```python
from build123d import *

# Parameters (mm, degrees)
CHAMFER1_SIZE = 0.5
FILLET1_R     = 10


with BuildPart() as part:
    # Sketch1 → Revolve1 (revolve)
    with BuildSketch(Plane(origin=(0, 0, 0), x_dir=(0, 0, -1), z_dir=(1, 0, 0)), mode=Mode.PRIVATE) as revolve1_sk:
        Polygon((0, 0), (0, -80), (11.00000000000001, -80), (11.00000000000001, -77), (2.5000000000000098, -77), (2.5000000000000098, -8), (1.4957064412197685, -8), (1.4957064412197685, -3.000000000000001), (2.500000000000019, -3.000000000000001), (2.500000000000019, -4e-16), align=None)
    revolve(revolve1_sk.sketch.rotate(Axis((0, 0, 0), (0, -1, 0)), 180), axis=Axis((0, 0, 0), (0, -1, 0)))

    # Chamfer1
    chamfer1_edges = [part.edges().sort_by_distance(p)[0] for p in [
        (-6.1e-16, -4e-16, -2.500000000000019),
    ]]
    chamfer(chamfer1_edges, length=CHAMFER1_SIZE)

    # Fillet1
    # the kernel refuses this fillet: 10 mm, written as the material it adds along each edge
    with BuildSketch(Plane(origin=(0, -77, 0), x_dir=(1.2e-16, 0, 1), z_dir=(1, 0, -1.2e-16))) as fillet1_piece_1:
        with BuildLine():
            CenterArc((12.500000000000007, -9.886859966642888), FILLET1_R, 98.62692655867836, 81.37307344132165)
            Line((11.000000000000053, -2.8422e-13), (10.970000000000054, 0.19773719933256473))
            ThreePointArc((10.970000000000054, 0.19773719933256473), (6.750000000000032, 0.20000000000000284), (2.5000000000000098, 0.20000000000000284))
            Line((2.5000000000000098, 0.20000000000000284), (2.3000000000000096, 0))
            Line((2.3000000000000096, 0), (2.300000000000007, -9.886859966642888))
            Line((2.300000000000007, -9.886859966642888), (2.500000000000007, -9.886859966642888))
        make_face()
    revolve(axis=Axis((0, -77, 0), (0, -1, 0)))


solid = part.part
```
Can you work these out from the model? Positions are in its coordinate system, mm. A direction names the side the tool comes from. Coordinates: 2 decimals unless noted, no trailing zeros. Order: outer loops, then holes, each group sorted by start corner. A loop starts at its lowest first (then second) coordinate and runs counter-clockwise, first axis right, second up.
1. I'm going to push flat-ended pins straight in: pin 1 (12 mm diameter, centred on y = -56.5, z = 0, fed in from -X); pin 2 (10 mm diameter, centred on x = -0.5, z = -8.5, fed in from +Y); pin 3 (6 mm diameter, centred on y = -69.5, z = -8, fed in from +X); pin 4 (4 mm diameter, centred on y = -34, z = -1.5, fed in from +X). Where does each tip first touch, or does it pass through?
2. Thinking about a two-plate mould opening in Y: for faces 1 (the face through (0, -80, 0)), 2 (the face through (-1.69, -1.73, -1.84)), 3 (the face through (2, -8, 0)), which applies, +Y half, -Y half, draft (parallel to the pull), parting line (faces both ways), or undercut?
3. I need wall thicknesses on line 1 (Y direction, x = 0, z = -1.75); line 2 (X direction, y = -23, z = -0.25); line 3 (Y direction, x = 6.5, z = -6.5). Which ranges of each line are inside material? Lowest first, please.
4. If we section it at B-B (x = 0): Please give me the cut outline in (y, z).
5. If we section it at A-A (z = 0): Please give me the cut outline in (x, y), then the cut area to 3 significant figures.
6. If we section it at D-D (y = -74.5): Please give me the cut outline in (x, z), then the cut area to 3 significant figures.
7. If we section it at C-C (y = -6): Please give me the cut outline in (x, z).
8. For faces 4 (the face through (0, 0, 0)), 5 (the face through (1.46, -5.46, -0.32)), 6 (the face through (2.44, -37.14, -0.54)), which set-ups out of +Z, -Z, +X, -X, +Y, -Y let a thin tool reach every point of the face, with its end or its side?
Entries:
1. pin 1: stops at x = -2.5
1. pin 2: stops at y = -71.5
1. pin 3: passes through
1. pin 4: stops at x = 2.5
2. face 1: -Y half
2. face 2: draft
2. face 3: undercut
3. line 1: y = -80 to -8, -3 to 0
3. line 2: x = -2.49 to 2.49
3. line 3: y = -80 to -76.55
4. outline: (-80, -11) - (-77, -11) arc R10 cw to (-67.11, -2.5) - (-8, -2.5) - (-8, -1.5) - (-3, -1.5) - (-3, -2.5) - (-0.5, -2.5) - (0, -2) - (0, 2) - (-0.5, 2.5) - (-3, 2.5) - (-3, 1.5) - (-8, 1.5) - (-8, 2.5) - (-67.11, 2.5) arc R10 cw to (-77, 11) - (-80, 11) - close
5. outline: (-11, -80) - (11, -80) - (11, -77) arc R10 cw to (2.5, -67.11) - (2.5, -8) - (1.5, -8) - (1.5, -3) - (2.5, -3) - (2.5, -0.5) - (2, 0) - (-2, 0) - (-2.5, -0.5) - (-2.5, -3) - (-1.5, -3) - (-1.5, -8) - (-2.5, -8) - (-2.5, -67.11) arc R10 cw to (-11, -77) - close
5. area: 482 mm2
6. outline: circle Ø11.52 at (0, 0)
6. area: 104 mm2
7. outline: circle Ø2.99 at (0, 0)
8. face 4: +Z, -Z, +X, -X, +Y
8. face 5: none
8. face 6: +Y
